Source: three-view drawing plus pictorial views. Frame: mm from the lowest corner of the part. Round coordinates to 2 decimals unless told otherwise and drop trailing zeros. Write each loop counter-clockwise with the first axis right and the second up, starting at its lowest first coordinate (ties: lowest second). Pieces come first, ordered by that corner, then holes. Notation, with made-up numbers: (33, 12.25) - (53, 12.25) arc R20 ccw to (53, 17.25) - close; hole circle Ø9 at (-33.5, -22.75). An arc over 180 degrees is marked (long way). Write each question's results on one line, items separated by ' | '.
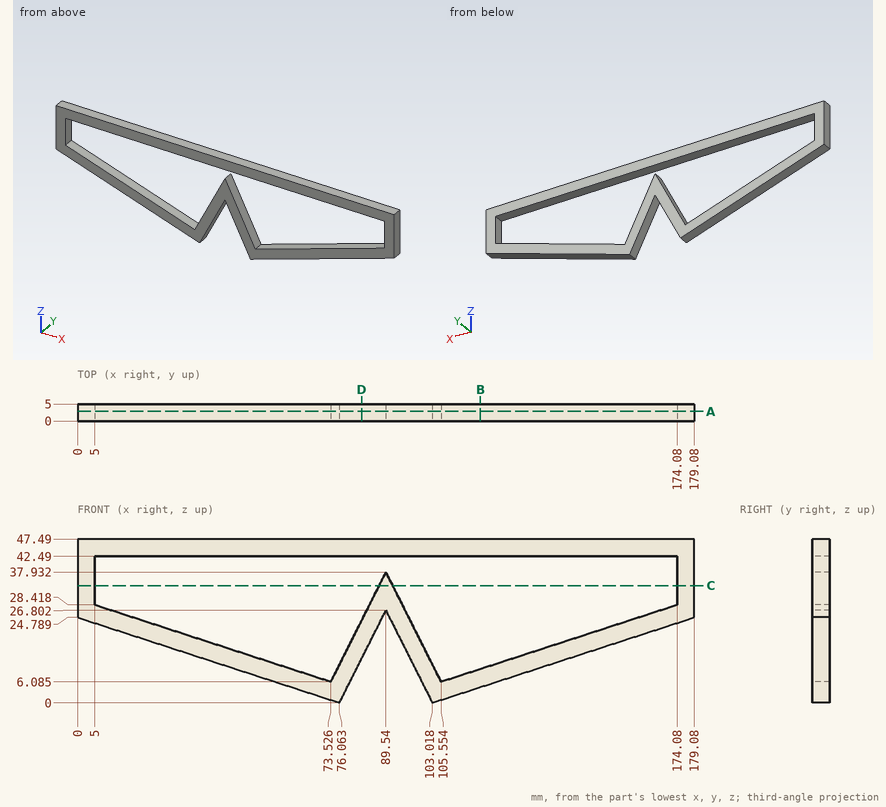
Q1. Section query D-D, the plane x = 82.5. Return loops of the section in (y, z).
Answer block:
outline: (0, 12.8) - (5, 12.8) - (5, 23.93) - (0, 23.93) - close; (0, 42.49) - (5, 42.49) - (5, 47.49) - (0, 47.49) - close
Q2. Section query B-B, the plane x = 117. Return loops of the section in (y, z) (1 decimal), plus the area to 3 significant figures.
Answer block:
outline: (0, 4.6) - (5, 4.6) - (5, 9.8) - (0, 9.8) - close; (0, 42.5) - (5, 42.5) - (5, 47.5) - (0, 47.5) - close | area: 51.3 mm2
Q3. Ray query, line 1 along X through (y, z) = (3.9, 36); line 2 along X through (y, z) = (1.55, 37.5) (1 decimal); line 3 along X through (y, z) = (3.15, 40). Return the intervals inside material, ascending.
Answer block:
line 1: 0 to 5, 88.57 to 90.51, 174.08 to 179.08 | line 2: 0 to 5, 89.3 to 89.8, 174.1 to 179.1 | line 3: 0 to 5, 174.08 to 179.08
Q4. Section query C-C, the plane z = 34. Return loops of the section in (x, y).
Answer block:
outline: (0, 0) - (5, 0) - (5, 5) - (0, 5) - close; (87.56, 0) - (91.52, 0) - (91.52, 5) - (87.56, 5) - close; (174.08, 0) - (179.08, 0) - (179.08, 5) - (174.08, 5) - close
Q5. Pin query (flat end, axial travel): pin 1 (1 mm diameter, centred on x = 123.5, y = 3, fed in from -Z). Return the tip coordinate at first contact, or that it passes through.
Answer block:
pin 1: z = 6.51
Q6. Section query A-A, the plane y = 2.85. Return loops of the section in (x, z) (1 decimal), plus the area to 3 significant figures.
Answer block:
outline: (0, 24.8) - (76.1, 0) - (89.5, 26.8) - (103, 0) - (179.1, 24.8) - (179.1, 47.5) - (0, 47.5) - close; hole (5, 28.4) - (73.5, 6.1) - (89.5, 37.9) - (105.6, 6.1) - (174.1, 28.4) - (174.1, 42.5) - (5, 42.5) - close | area: 2,140 mm2
